from build123d import *

# Parameters (mm, degrees)
BOSS_EXTRUDE1_DEPTH      = 20
CUT_EXTRUDE1_DEPTH       = 3
SKETCH4_W                = 3
SKETCH4_H                = 17
BOSS_EXTRUDE2_DEPTH      = 14
SKETCH6_W                = 3
SKETCH6_H                = 17
BOSS_EXTRUDE3_DEPTH      = 7.5
SKETCH7_R                = 1.5
CUT_EXTRUDE3_DEPTH       = 7.5
SKETCH8_R                = 1.5
CUT_EXTRUDE4_DEPTH       = 10
SKETCH10_R               = 3
CUT_EXTRUDE6_DEPTH       = 8
BOSS_EXTRUDE4_DEPTH      = 2
BOSS_EXTRUDE4_DEPTH_BACK = 2
SKETCH12_W               = 14
SKETCH12_H               = 17
BOSS_EXTRUDE5_DEPTH      = 2
BOSS_EXTRUDE6_DEPTH      = 2
BOSS_EXTRUDE7_DEPTH      = 20


with BuildPart() as part:
    # Sketch1 → Boss-Extrude1 (new body)
    with BuildSketch(Plane.XY):
        with BuildLine():
            Line((-3, -6), (-3, -40.891511))
            Line((-3, -40.891511), (0, -40.891511))
            Line((0, -40.891511), (0, -3))
            ThreePointArc((0, -3), (-0.878679656, -0.878679656), (-3, 0))
            Line((-3, 0), (-27.084538342, 0))
            ThreePointArc((-27.084538342, 0), (-29.205858686, 0.878679656), (-30.084538342, 3))
            Line((-30.084538342, 3), (-30.084538342, 31.8))
            Line((-30.084538342, 31.8), (-33.084538342, 31.8))
            Line((-33.084538342, 31.8), (-33.084538342, 0))
            ThreePointArc((-33.084538342, 0), (-32.205858686, -2.121320344), (-30.084538342, -3))
            Line((-30.084538342, -3), (-6, -3))
            ThreePointArc((-6, -3), (-3.878679656, -3.878679656), (-3, -6))
        make_face()
    extrude(amount=BOSS_EXTRUDE1_DEPTH)

    # Sketch2 → Cut-Extrude1 (cut)
    with BuildSketch(Plane(origin=(-30.084538342, 0, 0), x_dir=(0, 0, -1), z_dir=(1, 0, 0))):
        with BuildLine():
            ThreePointArc((-10, 31.8), (-2.928932188, 28.871067812), (0, 21.8))
            Line((0, 21.8), (0, 31.8))
            Line((0, 31.8), (-10, 31.8))
        make_face()
        with BuildLine():
            ThreePointArc((-20, 21.8), (-17.071067812, 28.871067812), (-10, 31.8))
            Line((-10, 31.8), (-20, 31.8))
            Line((-20, 31.8), (-20, 21.8))
        make_face()
    extrude(amount=-CUT_EXTRUDE1_DEPTH, mode=Mode.SUBTRACT)

    # Sketch4 → Boss-Extrude2 (add)
    with BuildSketch(Plane.XY.offset(20)):
        with Locations((-31.584538342, 13.3)):
            Rectangle(SKETCH4_W, SKETCH4_H)
    extrude(amount=BOSS_EXTRUDE2_DEPTH)

    # Sketch6 → Boss-Extrude3 (add)
    with BuildSketch(Plane.ZY.offset(33.084538342)):
        with Locations((32.5, 13.3)):
            Rectangle(SKETCH6_W, SKETCH6_H)
    extrude(amount=BOSS_EXTRUDE3_DEPTH)

    # Sketch7 → Cut-Extrude3 (cut)
    with BuildSketch(Plane(origin=(0, 0, 31), x_dir=(-1, 0, 0), z_dir=(0, 0, -1))):
        with Locations(Location((34.084538342, 18.8, 0), (0, 0, 131.810314896))):
            Circle(SKETCH7_R)
        with Locations(Location((34.084538342, 7.3, 0), (0, 0, 131.810314896))):
            Circle(SKETCH7_R)
    extrude(amount=-CUT_EXTRUDE3_DEPTH, mode=Mode.SUBTRACT)

    # Sketch8 → Cut-Extrude4 (cut)
    with BuildSketch(Plane.ZY.offset(33.084538342)):
        with Locations(Location((10, 21.8, 0), (0, 0, 270))):
            Circle(SKETCH8_R)
    extrude(amount=-CUT_EXTRUDE4_DEPTH, mode=Mode.SUBTRACT)

    # Sketch10 → Cut-Extrude6 (cut)
    with BuildSketch(Plane(origin=(0, 0, 31), x_dir=(-1, 0, 0), z_dir=(0, 0, -1))):
        with Locations((34.084538342, 7.3)):
            Circle(SKETCH10_R)
        with Locations((34.084538342, 18.8)):
            Circle(SKETCH10_R)
    extrude(amount=CUT_EXTRUDE6_DEPTH, mode=Mode.SUBTRACT)

    # Sketch11 → Boss-Extrude4 (add, two sides: drawn at the far end of the back side and taken through both)
    with BuildSketch(Plane(origin=(0, 13.3, 0), x_dir=(1, 0, 0), z_dir=(0, 1, 0)).offset(-BOSS_EXTRUDE4_DEPTH_BACK)):
        Polygon((-33.084538342, -25.5), (-33.084538342, -31), (-40.584538342, -31), align=None)
    extrude(amount=BOSS_EXTRUDE4_DEPTH + BOSS_EXTRUDE4_DEPTH_BACK)

    # Sketch12 → Boss-Extrude5 (add)
    with BuildSketch(Plane(origin=(-30.084538342, 0, 0), x_dir=(0, 0, -1), z_dir=(1, 0, 0))):
        with Locations((-27, 13.3)):
            Rectangle(SKETCH12_W, SKETCH12_H)
    extrude(amount=BOSS_EXTRUDE5_DEPTH)

    # Sketch15 → Boss-Extrude6 (add)
    with BuildSketch(Plane(origin=(-30.084538342, 0, 0), x_dir=(0, 0, -1), z_dir=(1, 0, 0))):
        with BuildLine():
            Line((0, 21.8), (0, 0))
            Line((0, 0), (-20, 0))
            Line((-20, 0), (-20, 21.8))
            ThreePointArc((-20, 21.8), (-10, 11.8), (0, 21.8))
        make_face()
    extrude(amount=BOSS_EXTRUDE6_DEPTH)

    # Sketch16 → Boss-Extrude7 (add)
    with BuildSketch(Plane(origin=(0, 0, 0), x_dir=(-1, 0, 0), z_dir=(0, 0, -1))):
        with BuildLine():
            Line((28.084538342, 0), (23.084538342, 0))
            ThreePointArc((23.084538342, 0), (26.620072248, 1.464466094), (28.084538342, 5))
            Line((28.084538342, 5), (28.084538342, 0))
        make_face()
    extrude(amount=-BOSS_EXTRUDE7_DEPTH)


solid = part.part
Check sheet for the modelled part. Datum: model origin and axes. Units: mm. A direction names the side the tool comes from. Round coordinates to 2 decimals unless told otherwise and drop trailing zeros. Order: outer loops, then holes, each group sorted by start corner. A loop starts at its lowest first (then second) coordinate and runs counter-clockwise, first axis right, second up.
Q1. Cross-section at B-B, the plane x = -29. Enter the section's corners in (y, z), plus the area to 3 significant figures.
Filled sheet:
outline: (-3, 0) - (21.8, 0) arc R10 cw to (21.8, 20) - (21.8, 34) - (4.8, 34) - (4.8, 20) - (-3, 20) - close
area: 577 mm2
Q2. Cross-section at D-D, the plane y = 18.8. Enter the section's corners in (x, z), plus the area to 3 significant figures.
Filled sheet:
outline: (-40.58, 31) - (-35.58, 31) - (-35.58, 34) - (-40.58, 34) - close; (-33.08, 0) - (-28.08, 0) - (-28.08, 0.46) - (-30.08, 0.46) - (-30.08, 19.54) - (-28.08, 19.54) - (-28.08, 34) - (-32.58, 34) - (-32.58, 31) - (-31.08, 31) - (-31.08, 23) - (-33.08, 23) - close
area: 129 mm2
Q3. Scan lines: L1, parallel to X at y = 18.8, z = 33.4; L2, parallel to Z at x = -29.5, y = 2.5; L3, parallel to X at y = 5, z = 7. Record each from-to range of solid material in increasing order.
Filled sheet:
L1: x = -40.58 to -35.58, -32.58 to -28.08
L2: z = 0 to 20
L3: x = -33.08 to -28.08
Q4. Cross-section at C-C, the plane z = 6. Enter the section's corners in (x, y).
Filled sheet:
outline: (-33.08, 0) arc R3 ccw to (-30.08, -3) - (-6, -3) arc R3 cw to (-3, -6) - (-3, -40.89) - (0, -40.89) - (0, -3) arc R3 ccw to (-3, 0) - (-23.08, 0) arc R5 cw to (-28.08, 5) - (-28.08, 12.63) - (-30.08, 12.63) - (-30.08, 30.97) - (-33.08, 30.97) - close
Q5. Depth check by flat-ended pin: P1, Ø1.6, axis at x = -37, z = 27.5, coming from the -Y side; P2, Ø6, axis at x = -37, z = 27, coming from the +Y side; P3, Ø2.5, axis at x = -34.08, y = 7.3, coming from the +Z side. Enter the tip coordinate at first touch or a pass-through.
Filled sheet:
P1: stops at y = 11.3
P2: stops at y = 15.3
P3: stops at z = 23
Q6. Draft check along Y on faces 1 (the face through (-32, 19, 23)), 2 (the face through (-13, 0, 10)), 3 (the face through (-3.9, -3.86, 9.86)), 4 (the face through (-34, 13, 34)). Enter one of: pulls with the +Y half, pulls with the -Y half, needs draft (parallel to the pull), parting line crosses it, or undercut.
Filled sheet:
face 1: undercut
face 2: pulls with the +Y half
face 3: pulls with the -Y half
face 4: needs draft
Q7. Cross-section at A-A, the plane y = 7.3. Enter the section's corners in (x, z), plus the area to 4 significant figures.
Filled sheet:
outline: (-40.58, 31) - (-35.58, 31) - (-35.58, 34) - (-40.58, 34) - close; (-33.08, 0) - (-28.08, 0) - (-28.08, 34) - (-32.58, 34) - (-32.58, 31) - (-31.08, 31) - (-31.08, 23) - (-33.08, 23) - close
area: 167.5 mm2
Q8. Set-up check for faces 5 (the face through (-35.56, 7.02, 32.48)), 6 (the face through (-28.085, 12, 21)), 7 (the face through (-29.1, 11.8, 10.2)), 8 (the face through (-37, 19, 31)), 9 (the face through (-32, 21.8, 29)): record each of +Z, -Z, +X, -X, +Y, -Y from which the full face is reachable in a straight line by a thin tool's end or side.
Filled sheet:
face 5: +Z
face 6: +Z, -Z, +X, +Y
face 7: +X, +Y
face 8: -X
face 9: +Z, +X, -X, +Y
